from build123d import *

# Parameters (mm, degrees)
F0_W     = 75.57
F0_H     = 22.6
F1_DEPTH = 2
F0_W_2   = 5
F0_H_2   = 20
F2_DEPTH = 11
F4_DEPTH = 75.57
F6_DEPTH = 25


with BuildPart() as f1:
    # F0 (on Top) → F1 (new body)
    with BuildSketch(Plane.XY):
        with Locations((37.785, -11.3)):
            Rectangle(F0_W, F0_H)
    extrude(amount=F1_DEPTH)

    # F0 (on Top) → F2 (join)
    with BuildSketch(Plane.XY):
        Polygon((35.285, 5), (-5, 5), (-5, -27.6), (80.57, -27.6), (80.57, 5), (40.285, 5), align=None)
        with Locations((37.785, -11.3)):
            Rectangle(F0_W, F0_H, mode=Mode.SUBTRACT)
        with Locations((37.785, 15)):
            Rectangle(F0_W_2, F0_H_2)
    extrude(amount=F2_DEPTH)

    # F3 (on face) → F4 (join, through all)
    with BuildSketch(Plane(origin=(75.57, 0, 0), x_dir=(0, -1, 0), z_dir=(-1, 0, 0))):
        Polygon((22.6, 6), (0, 2), (22.6, 2), align=None)
    extrude(amount=F4_DEPTH)

    # F5 (on face) → F6 (cut)
    with BuildSketch(Plane.YZ.offset(40.285)):
        Polygon((5, 6.94435), (25, 2.385827), (25, 11), (5, 11), align=None)
    extrude(amount=-F6_DEPTH, mode=Mode.SUBTRACT)


solid = f1.part
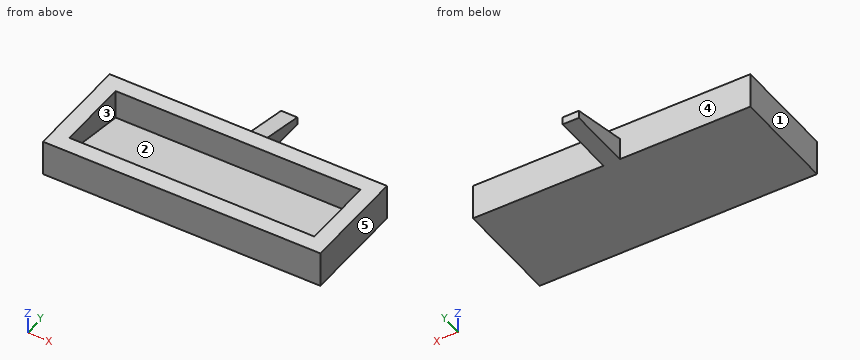
Can you work these out from the model? Positions are in its coordinate system, mm. Face numbers are marked on the shaded views. A direction names the side the tool comes from. Coordinates: 2 decimals unless noted, no trailing zeros. Loops run counter-clockwise (first coordinate to the right, second up) from the corner with the lowest first, then second, coordinate; pieces in that order, holes last. Notation, with made-up numbers: M -25,71.5 L 5,71.5 A21 ccw 5,108.5 Z; hole C 2,10.25 d7. An arc over 180 degrees is marked long. Answer as CSV lines item,"result". Start each with the question number.
1. For the marked faces 1 and 2, which set-ups out of +Z, -Z, +X, -X, +Y, -Y let a thin tool reach every point of the face, with its end or its side?
2. Suppose I cut it at B-B, the plane z = 8.25. List the corners of the cut face in (x, y) for me, plus the area to 3 significant figures.
3. Suppose I cut it at D-D, the plane z = 3.5. List the corners of the cut face in (x, y) for me (3 decimals), plus the area to 3 significant figures.
4. Thinking about a two-plate mould opening in X: for the marked faces 3, 4 and 5, which applies, +X half, -X half, draft (parallel to the pull), parting line (faces both ways), or undercut?
5. Suppose I cut it at C-C, the plane y = -19. List the corners of the cut face in (x, z) for me.
6. For pin 1 Ø3.5 at (y, z) = (11.5, 5) entering from -X (3 decimals); pin 2 Ø1 at (x, y) = (12, -15.5) entering from +Z; pin 3 Ø6 at (x, z) = (28, 9.5) entering from +Y, each with a flat end and sliding along its axis, tell me the tip position at first contact or that it passes through.
7. If I drill on probe 1 along X at (y, z) = (-14, 6.25); probe 2 along Y at (x, z) = (62, 6.5); probe 3 along X at (y, z) = (10, 2) (3 decimals), over which ranges is the centre line in solid material (lowest first)? Write a range as [from, to].
8. Suppose I cut it at A-A, the plane x = 43.5. List the corners of the cut face in (y, z) for me.
Output:
1,face 1,"+Z, -Z, -X, +Y, -Y"
1,face 2,"+Z"
2,outline,"M -5,-27.6 L 80.57,-27.6 L 80.57,5 L -5,5 Z; hole M 0,-22.6 L 75.57,-22.6 L 75.57,0 L 0,0 Z"
2,area,"1,080 mm^2"
3,outline,"M -5,-27.6 L 80.57,-27.6 L 80.57,5 L 40.285,5 L 40.285,20.112 L 35.285,20.112 L 35.285,5 L -5,5 Z; hole M 0,-8.475 L 75.57,-8.475 L 75.57,0 L 0,0 Z"
3,area,"2,220 mm^2"
4,face 3,"undercut"
4,face 4,"draft"
4,face 5,"+X half"
5,outline,"M -5,0 L 80.57,0 L 80.57,11 L 75.57,11 L 75.57,5.36 L 0,5.36 L 0,11 L -5,11 Z"
6,pin 1,"stops at x = 35.285"
6,pin 2,"stops at z = 4.83"
6,pin 3,"stops at y = 5"
7,probe 1,"x = [-5, 0], [75.57, 80.57]"
7,probe 2,"y = [-27.6, -22.6], [0, 5]"
7,probe 3,"x = [35.285, 40.285]"
8,outline,"M -27.6,0 L 5,0 L 5,11 L 0,11 L 0,2 L -22.6,6 L -22.6,11 L -27.6,11 Z"
